Input: part model. Units: mm. Frame: model coordinates. Face numbers are marked on the shaded views. A direction names the side the tool comes from. Give positions to 0.01 mm unless a question says otherwise; leave off trailing zeros. Loops run counter-clockwise (first coordinate to the right, second up) from the corner with the lowest first, then second, coordinate; pieces in that order, holes last. Notation, with made-up numbers: (-40, 71.25) -> (-8, 71.25) arc R9 cw to (-8, 84.25) -> close; hole circle Ø10 at (47, -23.5). An arc over 180 degrees is marked (long way). Use CSV: the item, a comma, the result in double quotes.
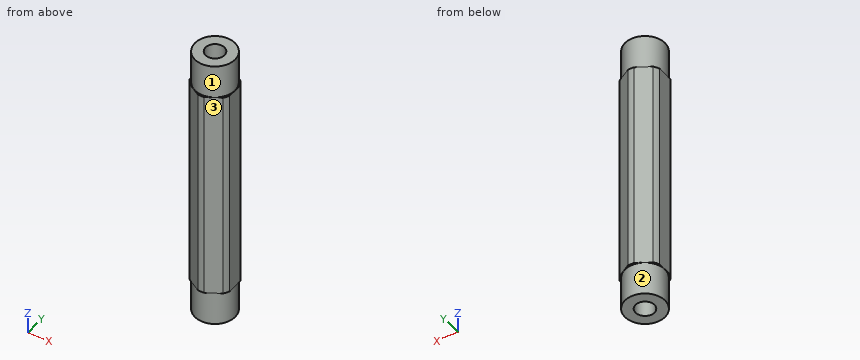
Autodesk Inventor part; units mm, degrees
ref_plane "YZ Plane" through (0, 0, 0) normal (1, 0, 0) x (0, 1, 0)
ref_plane "XZ Plane" through (0, 0, 0) normal (0, 1, 0) x (-1, 0, 0)
ref_plane "XY Plane" through (0, 0, 0) normal (0, 0, 1) x (1, 0, 0)
sketch "Sketch1" plane through (0, 0, 0) normal (0, 0, 1) x (1, 0, 0)
  line L0 (-4.7625, -2.7496) -> (-4.7625, 2.7496)
  line L1 (-4.7625, 2.7496) -> (0, 5.4993)
  line L2 (0, 5.4993) -> (4.7625, 2.7496)
  line L3 (4.7625, 2.7496) -> (4.7625, -2.7496)
  line L4 (4.7625, -2.7496) -> (0, -5.4993)
  line L5 (0, -5.4993) -> (-4.7625, -2.7496)
  point P0 (0, 0)
  point P1 (0, 0)
  dimension "Size" = 9.525
extrude "Extrusion1" add sketch "Sketch1" along normal mid plane 66.675
sketch "Sketch3" plane through (0, 0, 33.3375) normal (0, 0, 1) x (1, 0, 0)
  line L0 (-4.7625, 2.7496) -> (0, 5.4993) construction
  line L1 (0, 5.4993) -> (4.7625, 2.7496) construction
  line L2 (4.7625, 2.7496) -> (4.7625, -2.7496) construction
  line L3 (4.7625, -2.7496) -> (0, -5.4993) construction
  line L4 (0, -5.4993) -> (-4.7625, -2.7496) construction
  line L5 (-4.7625, -2.7496) -> (-4.7625, 2.7496) construction
  point P0 (0, 0)
hole "Hole1" at (0, 0, 33.3375) direction (0, 0, -1) diameter 4.4958 end through all
sketch "Sketch4" plane through (0, 0, 33.3375) normal (0, 0, 1) x (1, 0, 0)
  circle A0 centre (0, 0) radius 2.2479 construction
  line L0 (-4.7625, 2.7496) -> (0, 5.4993) construction
  line L1 (0, 5.4993) -> (4.7625, 2.7496) construction
  line L2 (4.7625, 2.7496) -> (4.7625, -2.7496) construction
  line L3 (4.7625, -2.7496) -> (0, -5.4993) construction
  line L4 (0, -5.4993) -> (-4.7625, -2.7496) construction
  line L5 (-4.7625, -2.7496) -> (-4.7625, 2.7496) construction
  circle A1 centre (0, 0) radius 5.1245
  circle A2 centre (0, 0) radius 8.89
  dimension "thunder" = 10.2489
  dimension "d16" = 17.78
extrude "Extrusion3" cut sketch "Sketch4" against normal through all
sketch "Sketch5" plane through (0, 0, -33.3375) normal (0, 0, -1) x (-1, 0, 0)
  arc A0 (-4.7625, -1.8917) -> (-4.0195, -3.1786) centre (0, 0) ccw
  line L0 (-4.0195, -3.1786) -> (-0.743, -5.0703)
  arc A1 (-0.743, -5.0703) -> (0.743, -5.0703) centre (0, 0) ccw
  line L1 (0.743, -5.0703) -> (4.0195, -3.1786)
  arc A2 (4.0195, -3.1786) -> (4.7625, -1.8917) centre (0, 0) ccw
  line L2 (4.7625, -1.8917) -> (4.7625, 1.8917)
  arc A3 (4.7625, 1.8917) -> (4.0195, 3.1786) centre (0, 0) ccw
  line L3 (4.0195, 3.1786) -> (0.743, 5.0703)
  arc A4 (0.743, 5.0703) -> (-0.743, 5.0703) centre (0, 0) ccw
  line L4 (-0.743, 5.0703) -> (-4.0195, 3.1786)
  arc A5 (-4.0195, 3.1786) -> (-4.7625, 1.8917) centre (0, 0) ccw
  line L5 (-4.7625, 1.8917) -> (-4.7625, -1.8917)
  circle A6 centre (0, 0) radius 2.2479
  circle A7 centre (0, 0) radius 2.2479 construction
  circle A8 centre (0, 0) radius 4.7625
  point P0 (-4.7625, 0)
  point P1 (-2.3813, 4.1244)
  point P2 (2.3813, 4.1244)
  point P3 (4.7625, 0)
  point P4 (2.3812, -4.1244)
  point P5 (-2.3812, -4.1244)
  dimension "d19" = 9.525
extrude "Extrusion4" cut sketch "Sketch5" against normal blind 8.001 contours L5 A8 L0 A0 | L5 A5 L4 A8 | A8 L1 A1 L0 | L4 A4 L3 A8 | A8 L2 A2 L1 | L3 A3 L2 A8
mirror "Mirror2" about plane through (0, 0, 0) normal (0, 0, 1) of "Extrusion4"
equation "\"bearing\" = 25.4"
properties part number "GP6-008" material "Aluminum 6061"
1) Section query C-C (z = -28). Return loops of the section in (x, y) (1 decimal).
From the geometry:
outline,"circle Ø9.5 at (0, 0); hole circle Ø4.5 at (0, 0)"
2) Contact query for flat-ended pins moving along their axis: pin 1 (4 mm diameter, centred on x = 0, y = 0, fed in from -Z); pin 2 (1 mm diameter, centred on y = -2.5, z = -14, fed in from -X). Output: stop coordinate, or through.
From the geometry:
pin 1,"passes through"
pin 2,"stops at x = -4.72"
3) Reachability of the marked faces 1, 2 and 3 from +Z, -Z, +X, -X, +Y, -Y: full face, straight path, thin tool, end or side. Return the list, or none.
From the geometry:
face 1,"+Z"
face 2,"-Z"
face 3,"+Z, -Z, +X, -Y"
4) Section query B-B (z = 4.5). Return loops of the section in (x, y), then the cut area to 3 significant figures.
From the geometry:
outline,"(-4.76, -1.89) arc R5.12 ccw to (-4.02, -3.18) -> (-0.74, -5.07) arc R5.12 ccw to (0.74, -5.07) -> (4.02, -3.18) arc R5.12 ccw to (4.76, -1.89) -> (4.76, 1.89) arc R5.12 ccw to (4.02, 3.18) -> (0.74, 5.07) arc R5.12 ccw to (-0.74, 5.07) -> (-4.02, 3.18) arc R5.12 ccw to (-4.76, 1.89) -> close; hole circle Ø4.5 at (0, 0)"
area,"61.1 mm^2"
5) Ray query, line 1 (X direction, y = 0, z = 11); line 2 (Y direction, x = 1, z = 15.5); line 3 (Y direction, x = 1.5, z = 22.5). Return the intervals inside material, ascending.
From the geometry:
line 1,"x = -4.76 to -2.25, 2.25 to 4.76"
line 2,"y = -4.92 to -2.01, 2.01 to 4.92"
line 3,"y = -4.63 to -1.67, 1.67 to 4.63"
6) Section query A-A (x = 0). Return loops of the section in (y, z), then the cut area to 3 significant figures.
From the geometry:
outline,"(-5.12, -25.34) -> (-4.76, -25.34) -> (-4.76, -33.34) -> (-2.25, -33.34) -> (-2.25, 33.34) -> (-4.76, 33.34) -> (-4.76, 25.34) -> (-5.12, 25.34) -> close; (2.25, -33.34) -> (4.76, -33.34) -> (4.76, -25.34) -> (5.12, -25.34) -> (5.12, 25.34) -> (4.76, 25.34) -> (4.76, 33.34) -> (2.25, 33.34) -> close"
area,"372 mm^2"
